Can you work these out from the model? Positions are in its coordinate system, mm. Face numbers are marked on the shaded views. A direction names the side the tool comes from. Coordinates: 2 decimals unless noted, no trailing zeros. Order: outer loops, then holes, each group sorted by start corner. A loop starts at its lowest first (then second) coordinate and runs counter-clockwise, first axis right, second up. Notation, with made-up numbers: (60.5, -7.75) -> (116.5, -7.75) arc R15 ccw to (116.5, 13.25) -> close; hole circle Ø3 at (61, -38.5). An arc over 180 degrees is marked (long way). Answer as CSV lines item,"result".
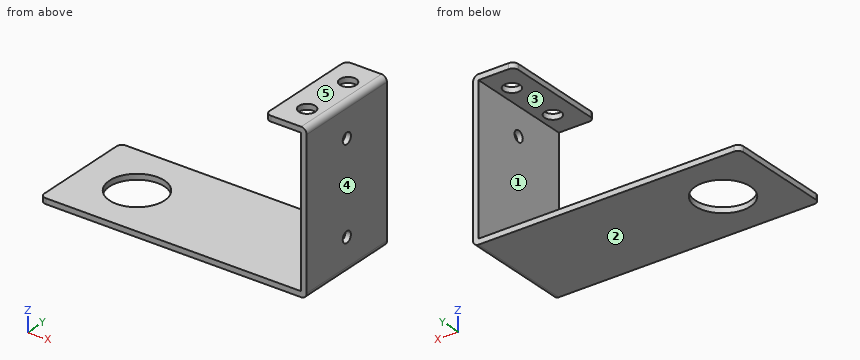
from build123d import *

# Parameters (mm, degrees)
SKETCH1_W           = 47.5
SKETCH1_H           = 19.6
SKETCH1_R           = 5
BOSS_EXTRUDE1_DEPTH = 1
BOSS_EXTRUDE2_START = -1
SKETCH2_W           = 1
SKETCH2_H           = 19.6
BOSS_EXTRUDE2_DEPTH = 28.512
SKETCH3_W           = 1
SKETCH3_H           = 19.6
BOSS_EXTRUDE3_DEPTH = 6.5
CUT_EXTRUDE1_REACH  = 30.512
SKETCH4_R           = 1.5
SKETCH6_R           = 1
CUT_EXTRUDE2_DEPTH  = 6.5
FILLET1_R           = 1


with BuildPart() as part:
    # Sketch1 → Boss-Extrude1 (new body)
    with BuildSketch(Plane.XY):
        Rectangle(SKETCH1_W, SKETCH1_H)
        with Locations((-13.45, 0)):
            Circle(SKETCH1_R, mode=Mode.SUBTRACT)
    extrude(amount=BOSS_EXTRUDE1_DEPTH)

    # Sketch2 → Boss-Extrude2 (add)
    with BuildSketch(Plane.XY.offset(1).offset(BOSS_EXTRUDE2_START)):
        with Locations((24.25, 0)):
            Rectangle(SKETCH2_W, SKETCH2_H)
    extrude(amount=BOSS_EXTRUDE2_DEPTH)

    # Sketch3 → Boss-Extrude3 (add)
    with BuildSketch(Plane.ZY.offset(-23.75)):
        with Locations((28.012, 0)):
            Rectangle(SKETCH3_W, SKETCH3_H)
    extrude(amount=BOSS_EXTRUDE3_DEPTH)

    # Sketch4 → Cut-Extrude1 (cut, up to next)
    with BuildSketch(Plane.XY.offset(28.512), mode=Mode.PRIVATE) as cut_extrude1_sk1:
        with Locations((21.25, 5)):
            Circle(SKETCH4_R)
    cut_extrude1_tool1 = extrude(cut_extrude1_sk1.sketch, amount=-CUT_EXTRUDE1_REACH, mode=Mode.PRIVATE) & part.part
    add(cut_extrude1_tool1.solids().sort_by_distance((21.25, 5, 28.512))[0], mode=Mode.SUBTRACT)
    # Sketch4 → Cut-Extrude1 (cut, up to next)
    with BuildSketch(Plane.XY.offset(28.512), mode=Mode.PRIVATE) as cut_extrude1_sk2:
        with Locations((21.25, -5)):
            Circle(SKETCH4_R)
    cut_extrude1_tool2 = extrude(cut_extrude1_sk2.sketch, amount=-CUT_EXTRUDE1_REACH, mode=Mode.PRIVATE) & part.part
    add(cut_extrude1_tool2.solids().sort_by_distance((21.25, -5, 28.512))[0], mode=Mode.SUBTRACT)

    # Sketch6 → Cut-Extrude2 (cut)
    with BuildSketch(Plane.ZY.offset(-23.75)):
        with Locations((6, 0)):
            Circle(SKETCH6_R)
        with Locations((22.512, 0)):
            Circle(SKETCH6_R)
    extrude(amount=-CUT_EXTRUDE2_DEPTH, mode=Mode.SUBTRACT)

    # Fillet1
    fillet1_edges = [part.edges().sort_by_distance(p)[0] for p in [
        (-23.75, 9.8, 0.5),
        (-23.75, -9.8, 0.5),
        (17.25, -9.8, 28.012),
        (17.25, 9.8, 28.012),
        (24.75, 0, 0),
        (24.75, 0, 28.512),
    ]]
    fillet(fillet1_edges, radius=FILLET1_R)


solid = part.part
Q1. We'd pull the mould along Z, two halves only. Please class the marked faces 3, 4 and 5: pulls with the +Z half, pulls with the -Z half, needs draft (parallel to the pull), parting line crosses it, or undercut.
Solution:
face 3,"undercut"
face 4,"needs draft"
face 5,"pulls with the +Z half"
Q2. If I drill on line 1 (Y direction, x = 21.25, z = 28.2); line 2 (Z direction, x = 20, y = -0.5); line 3 (Y direction, x = -13.45, z = 0.7), over which ranges is the centre line in solid material (lowest first)?
Solution:
line 1,"-9.8 to -6.5, -3.5 to 3.5, 6.5 to 9.8"
line 2,"0 to 1, 27.51 to 28.51"
line 3,"-9.8 to -5, 5 to 9.8"
Q3. Imagine slicing it at D-D (y = -7). List the corners of the cut face in (x, z) for me, and give its area (3 significant figures).
Solution:
outline,"(-23.75, 0) -> (23.75, 0) arc R1 ccw to (24.75, 1) -> (24.75, 27.51) arc R1 ccw to (23.75, 28.51) -> (17.25, 28.51) -> (17.25, 27.51) -> (23.75, 27.51) -> (23.75, 1) -> (-23.75, 1) -> close"
area,"82.1 mm2"
Q4. For P1, Ø4, axis at y = -5, z = 10.5, coming from the -X side; P2, Ø1.5, axis at x = 0.5, y = -6.5, coming from the +Z side; P3, Ø0.8, axis at y = -1.5, z = 28, coming from the -X side, each with a flat end and sliding along its axis, tell me the tip position at first contact or that it passes through.
Solution:
P1,"x = 23.75"
P2,"z = 1"
P3,"x = 17.25"
Q5. Which directions (+Z, -Z, +X, -X, +Y, -Y) give clear straight access to the entire face, cutting with the end or side of a thin tool? Please do the marked faces 1 and 2.
Solution:
face 1,"-X, +Y, -Y"
face 2,"-Z, +X, -X, +Y, -Y"
Q6. Imagine slicing it at C-C (x = -13.45). List the corners of the cut face in (y, z) for me, and give its area (3 significant figures).
Solution:
outline,"(-9.8, 0) -> (-5, 0) -> (-5, 1) -> (-9.8, 1) -> close; (5, 0) -> (9.8, 0) -> (9.8, 1) -> (5, 1) -> close"
area,"9.60 mm2"
Q7. Imagine slicing it at B-B (y = 0). List the corners of the cut face in (x, z) for me, and give its area (3 significant figures).
Solution:
outline,"(-23.75, 0) -> (-18.45, 0) -> (-18.45, 1) -> (-23.75, 1) -> close; (-8.45, 0) -> (23.75, 0) arc R1 ccw to (24.75, 1) -> (24.75, 5) -> (23.75, 5) -> (23.75, 1) -> (-8.45, 1) -> close; (17.25, 27.51) -> (23.75, 27.51) -> (23.75, 23.51) -> (24.75, 23.51) -> (24.75, 27.51) arc R1 ccw to (23.75, 28.51) -> (17.25, 28.51) -> close; (23.75, 7) -> (24.75, 7) -> (24.75, 21.51) -> (23.75, 21.51) -> close"
area,"68.1 mm2"
Q8. Imagine slicing it at A-A (x = 21.25). List the corners of the cut face in (y, z) for me.
Solution:
outline,"(-9.8, 0) -> (9.8, 0) -> (9.8, 1) -> (-9.8, 1) -> close; (-9.8, 27.51) -> (-6.5, 27.51) -> (-6.5, 28.51) -> (-9.8, 28.51) -> close; (-3.5, 27.51) -> (3.5, 27.51) -> (3.5, 28.51) -> (-3.5, 28.51) -> close; (6.5, 27.51) -> (9.8, 27.51) -> (9.8, 28.51) -> (6.5, 28.51) -> close"
